The model under review builds one solid part; all positions refer to its coordinate system, in mm. A direction names the side the tool comes from. Coordinates: 2 decimals unless noted, no trailing zeros. Order: outer loops, then holes, each group sorted by start corner. A loop starts at its lowest first (then second) coordinate and runs counter-clockwise, first axis right, second up.
```python
from build123d import *

# Parameters (mm, degrees)
SKETCH_1_R          = 10
SKETCH_1_R_2        = 1.5
SKETCH_1_R_3        = 4
EXTRUDE_1_DEPTH     = 6
SKETCH_2_R          = 5.15
CUT_EXTRUDE_1_DEPTH = 4


with BuildPart() as part:
    # Эскиз1 → Бобышка-Вытянуть1 (new body)
    with BuildSketch(Plane(origin=(0, 0, 0), x_dir=(1, 0, 0), z_dir=(0, 1, 0))):
        with Locations(Location((0, 0, 0), (0, 0, 270))):
            Circle(SKETCH_1_R)
        with Locations(Location((0, 7.5, 0), (0, 0, 270))):
            Circle(SKETCH_1_R_2, mode=Mode.SUBTRACT)
        with Locations(Location((0, -7.5, 0), (0, 0, 270))):
            Circle(SKETCH_1_R_2, mode=Mode.SUBTRACT)
        with Locations(Location((0, 0, 0), (0, 0, 270))):
            Circle(SKETCH_1_R_3, mode=Mode.SUBTRACT)
    extrude(amount=EXTRUDE_1_DEPTH)

    # Эскиз2 → Вырез-Вытянуть1 (cut)
    with BuildSketch(Plane(origin=(0, 6, 0), x_dir=(1, 0, 0), z_dir=(0, 1, 0))):
        with Locations(Location((0, 0, 0), (0, 0, 270))):
            Circle(SKETCH_2_R)
    extrude(amount=-CUT_EXTRUDE_1_DEPTH, mode=Mode.SUBTRACT)


solid = part.part
```
(1) We need section D-D, the plane z = -3. Write out the cut boundary in (x, y), and give its area (3 significant figures).
A:
outline: (-9.54, 0) - (-2.65, 0) - (-2.65, 2) - (-4.19, 2) - (-4.19, 6) - (-9.54, 6) - close; (2.65, 0) - (9.54, 0) - (9.54, 6) - (4.19, 6) - (4.19, 2) - (2.65, 2) - close
area: 70.4 mm2
(2) Draft analysis for pull direction X (two halves, no side actions). For faces 1 (the face through (-3, 2, 3)), 2 (the face through (2, 6, -5)), 3 (the face through (-3.905, 0.986, -0.867)), 4 (the face through (-9.76, 2.96, -2.17)), state which applies: released by +X, released by -X, zero draft, split by the parting line, or undercut.
A:
face 1: undercut
face 2: zero draft
face 3: undercut
face 4: split by the parting line
(3) For pin 1 Ø1 at (y, z) = (1.5, 1.5) entering from -X; pin 2 Ø1.5 at (y, z) = (2.5, -2.5) entering from -X; pin 3 Ø8 at (x, z) = (0, 0.5) entering from +Y, all flat-tipped, find the tip position at first contact; note any pin that passes through.
A:
pin 1: stops at x = -9.95
pin 2: stops at x = -9.85
pin 3: stops at y = 2
(4) We need section A-A, the plane x = 0. Write out the cut boundary in (y, z).
A:
outline: (0, -10) - (6, -10) - (6, -9) - (0, -9) - close; (0, -6) - (6, -6) - (6, -5.15) - (2, -5.15) - (2, -4) - (0, -4) - close; (0, 4) - (2, 4) - (2, 5.15) - (6, 5.15) - (6, 6) - (0, 6) - close; (0, 9) - (6, 9) - (6, 10) - (0, 10) - close
(5) Wall thickness on probe 1 along X at (y, z) = (1.05, 0); probe 2 along X at (y, z) = (3.9, 0); probe 3 along Z at (x, y) = (-0.75, 2.5): over which ranges is each line inside the solid? List them lowest first.
A:
probe 1: x = -10 to -4, 4 to 10
probe 2: x = -10 to -5.15, 5.15 to 10
probe 3: z = -9.97 to -8.8, -6.2 to -5.1, 5.1 to 6.2, 8.8 to 9.97
(6) Machinability: for faces 5 (the face through (-5.028, 4.028, -1.116)), 6 (the face through (0, 3, 6)), which of the approach directions +Z, -Z, +X, -X, +Y, -Y give a long, thin tool a straight path to every point of the face, cutting with its end or side? Answer none if there is none.
A:
face 5: +Y
face 6: +Y, -Y
(7) We need section C-C, the plane y = 0.8. Write out the cut boundary in (x, z), and give its area (3 significant figures).
A:
outline: circle Ø20 at (0, 0); hole circle Ø8 at (0, 0); hole circle Ø3 at (0, -7.5); hole circle Ø3 at (0, 7.5)
area: 250 mm2
(8) We need section B-B, the plane z = 0. Write out the cut boundary in (x, y).
A:
outline: (-10, 0) - (-4, 0) - (-4, 2) - (-5.15, 2) - (-5.15, 6) - (-10, 6) - close; (4, 0) - (10, 0) - (10, 6) - (5.15, 6) - (5.15, 2) - (4, 2) - close
